Autodesk Inventor part; units mm, degrees
ref_plane "YZ Plane" through (0, 0, 0) normal (1, 0, 0) x (0, 1, 0)
ref_plane "XZ Plane" through (0, 0, 0) normal (0, 1, 0) x (-1, 0, 0)
ref_plane "XY Plane" through (0, 0, 0) normal (0, 0, 1) x (1, 0, 0)
sketch "Sketch1" plane through (0, 0, 0) normal (0, 0, 1) x (1, 0, 0)
  line L0 (0, 0) -> (8, 0)
  line L1 (8, 0) -> (8, 8)
  line L2 (8, 8) -> (0, 8)
  line L3 (0, 8) -> (0, 0)
  line L4 (-3, 11) -> (11, 11)
  line L5 (11, 11) -> (11, -3)
  line L6 (11, -3) -> (-3, -3)
  line L7 (-3, -3) -> (-3, 11)
  dimension "d0" = 8
  dimension "d1" = 8
  dimension "d2" = 3
extrude "Extrusion1" add sketch "Sketch1" along normal blind 1.5 contours L3 L2 L1 L0 | L4 L5 L6 L7
extrude "Extrusion2" add sketch "Sketch1" against normal blind 4
chamfer "Chamfer1" distance 2.5 angle 45 4 edges at (8, 4, -4) (4, 0, -4) (4, 8, -4) (0, 4, -4)
sketch "Sketch2" plane through (0, 0, 0) normal (0, 0, -1) x (-1, 0, 0)
  line L0 (-8, 8) -> (-8, 0)
  line L1 (-8, 0) -> (0, 0)
  line L2 (0, 0) -> (0, 8)
  line L3 (0, 8) -> (-8, 8)
  point P0 (-4, 4)
hole "Hole1" at (4, 4, 0) direction (0, 0, 1) diameter 2 depth 8 tip angle 118
chamfer "Chamfer2" distance 2 angle 45 8 edges at (9.25, 9.25, -2.75) (-1.25, 9.25, -2.75) (-1.25, -1.25, -2.75) (9.25, -1.25, -2.75) (11, -3, -1.25) (11, 11, -1.25) (-3, -3, -1.25) (-3, 11, -1.25)
fillet "Fillet2" radius 1.5 8 edges at (11, 9, -1.25) (9, 11, -1.25) (11, -1, -1.25) (9, -3, -1.25) (-1, -3, -1.25) (-3, -1, -1.25) (-1, 11, -1.25) (-3, 9, -1.25)
properties part number "CNCM_ALU_Visual_inspection_tray_leg_holder" material "Aluminum 6061"
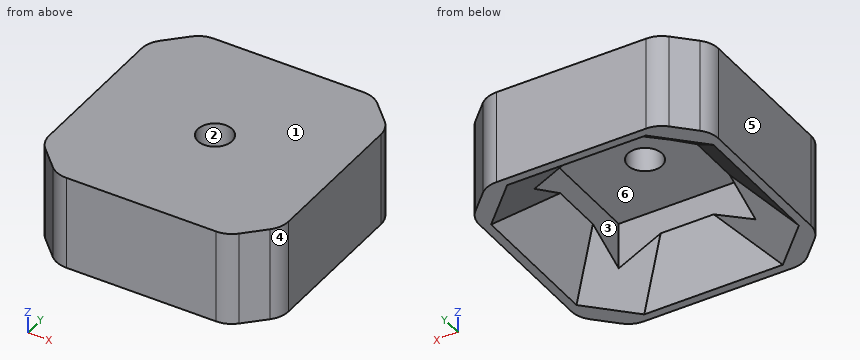
Source: CAD feature listing. Evaluate the final solid. Frame: model axes, mm. Face numbers are marked on the shaded views. A direction names the side the tool comes from. Round coordinates to 2 decimals unless told otherwise and drop trailing zeros. Loops run counter-clockwise (first coordinate to the right, second up) from the corner with the lowest first, then second, coordinate; pieces in that order, holes last.
(1) Access query for the marked faces 5 and 6. Directions: +Z, -Z, +X, -X, +Y, -Y. A direction counts if a zero-diameter tool reaches every point of the face in a straight line with its end or side. Return the directions, or none.
From the geometry:
face 5: +Z, -Z, -X, +Y, -Y
face 6: -Z
(2) Section query A-A (y = 4). Output: boundary loops of the cut face in (x, z).
From the geometry:
outline: (-3, -4) - (-2.5, -4) - (0, -1.5) - (0, 0) - (3, 0) - (3, 1.5) - (-3, 1.5) - close; (5, 0) - (8, 0) - (8, -1.5) - (10.5, -4) - (11, -4) - (11, 1.5) - (5, 1.5) - close
(3) Pull-direction query (X, two-part tool) for the marked faces 1, 2, 3 and 4; classes: +X half, -X half, draft (parallel to the pull), parting line (faces both ways), or undercut.
From the geometry:
face 1: draft
face 2: undercut
face 3: undercut
face 4: +X half
(4) Contact query for a flat-ended pin moving along its axis: pin 1 Ø6 at (x, y) = (5, 2) entering from -Z. Output: stop coordinate, or through.
From the geometry:
pin 1: stops at z = -2.5
(5) Section query D-D (z = -0.35). Output: boundary loops of the cut face in (x, y).
From the geometry:
outline: (-3, -0.38) arc R1.5 ccw to (-2.56, -1.44) - (-1.44, -2.56) arc R1.5 ccw to (-0.38, -3) - (8.38, -3) arc R1.5 ccw to (9.44, -2.56) - (10.56, -1.44) arc R1.5 ccw to (11, -0.38) - (11, 8.38) arc R1.5 ccw to (10.56, 9.44) - (9.44, 10.56) arc R1.5 ccw to (8.38, 11) - (-0.38, 11) arc R1.5 ccw to (-1.44, 10.56) - (-2.56, 9.44) arc R1.5 ccw to (-3, 8.38) - close; hole (0, 0) - (8, 0) - (8, 8) - (0, 8) - close
(6) Section query B-B (z = 1.1). Output: boundary loops of the cut face in (x, y), and give its area (3 significant figures).
From the geometry:
outline: (-3, -0.38) arc R1.5 ccw to (-2.56, -1.44) - (-1.44, -2.56) arc R1.5 ccw to (-0.38, -3) - (8.38, -3) arc R1.5 ccw to (9.44, -2.56) - (10.56, -1.44) arc R1.5 ccw to (11, -0.38) - (11, 8.38) arc R1.5 ccw to (10.56, 9.44) - (9.44, 10.56) arc R1.5 ccw to (8.38, 11) - (-0.38, 11) arc R1.5 ccw to (-1.44, 10.56) - (-2.56, 9.44) arc R1.5 ccw to (-3, 8.38) - close; hole circle Ø2 at (4, 4)
area: 184 mm2
(7) Material intervals for probe 1 along X at (y, z) = (4, 0.9); probe 2 along X at (y, z) = (2, -0.4), sorted ascending.
From the geometry:
probe 1: x = -3 to 3, 5 to 11
probe 2: x = -3 to 0, 8 to 11
